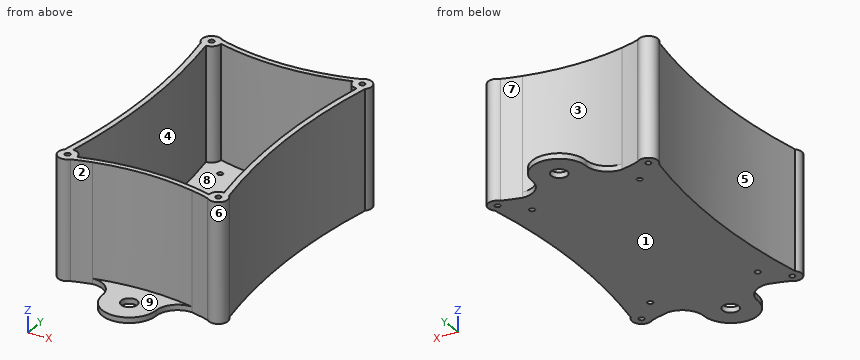
from build123d import *

# Parameters (mm, degrees)
F0_R     = 1
F1_DEPTH = 44
F0_R_2   = 3
F2_DEPTH = 2


with BuildPart() as f1:
    # F0 (on Top) → F1 (new body)
    with BuildSketch(Plane.XY):
        with BuildLine():
            ThreePointArc((-77.468398, 50.197146), (-73.493525, 8.17202), (-77.468398, -33.853106))
            ThreePointArc((-77.468398, -33.853106), (-77.468398, -38.802854), (-72.518651, -38.802854))
            ThreePointArc((-72.518651, -38.802854), (-68.996757, -37.763021), (-65.432755, -36.878214))
            ThreePointArc((-65.432755, -36.878214), (-46.993525, -34.82798), (-28.554295, -36.878214))
            ThreePointArc((-28.554295, -36.878214), (-24.990293, -37.763021), (-21.468398, -38.802854))
            ThreePointArc((-21.468398, -38.802854), (-16.518651, -38.802854), (-16.518651, -33.853106))
            ThreePointArc((-16.518651, -33.853106), (-20.493525, 8.17202), (-16.518651, 50.197146))
            ThreePointArc((-16.518651, 50.197146), (-16.518651, 55.146894), (-21.468398, 55.146894))
            ThreePointArc((-21.468398, 55.146894), (-24.990293, 54.10706), (-28.554295, 53.222254))
            ThreePointArc((-28.554295, 53.222254), (-46.993525, 51.17202), (-65.432755, 53.222254))
            ThreePointArc((-65.432755, 53.222254), (-68.996757, 54.10706), (-72.518651, 55.146894))
            ThreePointArc((-72.518651, 55.146894), (-77.468398, 55.146894), (-77.468398, 50.197146))
        make_face()
        with Locations((-74.993525, -36.32798)):
            Circle(F0_R, mode=Mode.SUBTRACT)
        with Locations((-18.993525, -36.32798)):
            Circle(F0_R, mode=Mode.SUBTRACT)
        with BuildLine():
            ThreePointArc((-74.993525, 49.17202), (-72.518651, 50.197146), (-71.493525, 52.67202))
            ThreePointArc((-71.493525, 52.67202), (-46.993525, 49.17202), (-22.493525, 52.67202))
            ThreePointArc((-22.493525, 52.67202), (-21.468398, 50.197146), (-18.993525, 49.17202))
            ThreePointArc((-18.993525, 49.17202), (-22.493525, 8.17202), (-18.993525, -32.82798))
            ThreePointArc((-18.993525, -32.82798), (-21.468398, -33.853106), (-22.493525, -36.32798))
            ThreePointArc((-22.493525, -36.32798), (-46.993525, -32.82798), (-71.493525, -36.32798))
            ThreePointArc((-71.493525, -36.32798), (-72.518651, -33.853106), (-74.993525, -32.82798))
            ThreePointArc((-74.993525, -32.82798), (-71.493525, 8.17202), (-74.993525, 49.17202))
        make_face(mode=Mode.SUBTRACT)
        with Locations((-74.993525, 52.67202)):
            Circle(F0_R, mode=Mode.SUBTRACT)
        with Locations((-18.993525, 52.67202)):
            Circle(F0_R, mode=Mode.SUBTRACT)
    extrude(amount=F1_DEPTH)

    # F0 (on Top) → F2 (join)
    with BuildSketch(Plane.XY):
        with BuildLine():
            ThreePointArc((-28.554295, -36.878214), (-46.993525, -34.82798), (-65.432755, -36.878214))
            ThreePointArc((-65.432755, -36.878214), (-59.507969, -39.04294), (-56.993525, -44.82798))
            ThreePointArc((-56.993525, -44.82798), (-46.993525, -54.82798), (-36.993525, -44.82798))
            ThreePointArc((-36.993525, -44.82798), (-34.47908, -39.04294), (-28.554295, -36.878214))
        make_face()
        with Locations((-46.993525, -44.82798)):
            Circle(F0_R_2, mode=Mode.SUBTRACT)
        with BuildLine():
            ThreePointArc((-56.993525, 61.17202), (-59.507969, 55.38698), (-65.432755, 53.222254))
            ThreePointArc((-65.432755, 53.222254), (-46.993525, 51.17202), (-28.554295, 53.222254))
            ThreePointArc((-28.554295, 53.222254), (-34.47908, 55.38698), (-36.993525, 61.17202))
            ThreePointArc((-36.993525, 61.17202), (-46.993525, 71.17202), (-56.993525, 61.17202))
        make_face()
        with Locations((-46.993525, 61.17202)):
            Circle(F0_R_2, mode=Mode.SUBTRACT)
        with BuildLine():
            ThreePointArc((-22.493525, 52.67202), (-46.993525, 49.17202), (-71.493525, 52.67202))
            ThreePointArc((-71.493525, 52.67202), (-72.518651, 50.197146), (-74.993525, 49.17202))
            ThreePointArc((-74.993525, 49.17202), (-71.493525, 8.17202), (-74.993525, -32.82798))
            ThreePointArc((-74.993525, -32.82798), (-72.518651, -33.853106), (-71.493525, -36.32798))
            ThreePointArc((-71.493525, -36.32798), (-46.993525, -32.82798), (-22.493525, -36.32798))
            ThreePointArc((-22.493525, -36.32798), (-21.468398, -33.853106), (-18.993525, -32.82798))
            ThreePointArc((-18.993525, -32.82798), (-22.493525, 8.17202), (-18.993525, 49.17202))
            ThreePointArc((-18.993525, 49.17202), (-21.468398, 50.197146), (-22.493525, 52.67202))
        make_face()
        with Locations((-66.993525, -28.32798)):
            Circle(F0_R, mode=Mode.SUBTRACT)
        with Locations((-26.993525, -28.32798)):
            Circle(F0_R, mode=Mode.SUBTRACT)
        with Locations((-66.993525, 44.67202)):
            Circle(F0_R, mode=Mode.SUBTRACT)
        with Locations((-26.993525, 44.67202)):
            Circle(F0_R, mode=Mode.SUBTRACT)
    extrude(amount=F2_DEPTH)


solid = f1.part
Source: CAD feature listing. Evaluate the final solid. Frame: model axes, mm. Face numbers are marked on the shaded views. A direction names the side the tool comes from. Round coordinates to 2 decimals unless told otherwise and drop trailing zeros. Loops run counter-clockwise (first coordinate to the right, second up) from the corner with the lowest first, then second, coordinate; pieces in that order, holes last. Notation, with made-up numbers: (65, 12) - (69, 12) arc R37 ccw to (69, 48) - close; hole circle Ø8 at (83.5, 35). An arc over 180 degrees is marked (long way). Write item = value, one per line. Start each with the question number.
Item 1: Section query C-C on y = 1.5. Output: boundary loops of the cut face in (x, z), plus the area to 3 significant figures.
Item 2: First-contact query: pin 1 Ø1 at (x, z) = (-34, 39) entering from -Y; pin 2 Ø10 at (x, z) = (-48.5, 32) entering from +Y; pin 3 Ø5 at (x, z) = (-25.5, 32) entering from -Y. Flat tips, straight axial feed; report the tip coordinate or a pass-through.
Item 3: Section query D-D on x = -39. Output: boundary loops of the cut face in (y, z), plus the area to 3 significant figures.
Item 4: Mould query, pull axis Y, two halves, no side actions, for the marked faces 1, 2, 3 and 4. Classes: released by +Y, released by -Y, zero draft, split by the parting line, or undercut.
Item 5: Reachability of the marked faces 5, 6, 7, 8 and 9 from +Z, -Z, +X, -X, +Y, -Y: full face, straight path, thin tool, end or side. Return the list, or none.
Item 6: Section query B-B on z = 16.5. Output: boundary loops of the cut face in (x, y), plus the area to 3 significant figures.
Item 7: Section query A-A on x = -47. Output: boundary loops of the cut face in (y, z), plus the area to 3 significant figures.
Item 8: Material intervals for line 1 (Y direction, x = -46.5, z = 21.5); line 2 (X direction, y = 9, z = 9.5); line 3 (Z direction, x = -52.5, y = 27.5), sorted ascending.
Results list:
q1.outline = (-73.59, 0) - (-20.39, 0) - (-20.39, 44) - (-22.4, 44) - (-22.4, 2) - (-71.59, 2) - (-71.59, 44) - (-73.59, 44) - close
q1.area = 275 mm²
q2.pin_1 = -35.92
q2.pin_2 = 51.42
q2.pin_3 = -38.33
q3.outline = (-50.84, 0) - (67.18, 0) - (67.18, 2) - (51.55, 2) - (51.55, 44) - (49.54, 44) - (49.54, 2) - (-33.19, 2) - (-33.19, 44) - (-35.21, 44) - (-35.21, 2) - (-50.84, 2) - close
q3.area = 405 mm²
q4.face_1 = zero draft
q4.face_2 = released by -Y
q4.face_3 = released by +Y
q4.face_4 = undercut
q5.face_5 = +Z, -Z, -X
q5.face_6 = +Z, -Z
q5.face_7 = +Z, -Z, +Y
q5.face_8 = +Z
q5.face_9 = +Z, -Y
q6.outline = (-77.47, -33.85) arc R3.5 ccw to (-72.52, -38.8) arc R83.94 cw to (-65.43, -36.88) arc R83.94 cw to (-28.55, -36.88) arc R83.94 cw to (-21.47, -38.8) arc R3.5 ccw to (-16.52, -33.85) arc R224.15 cw to (-16.52, 50.2) arc R3.5 ccw to (-21.47, 55.15) arc R83.94 cw to (-28.55, 53.22) arc R83.94 cw to (-65.43, 53.22) arc R83.94 cw to (-72.52, 55.15) arc R3.5 ccw to (-77.47, 50.2) arc R224.15 cw to start; hole circle Ø2 at (-74.99, -36.33); hole circle Ø2 at (-74.99, 52.67); hole (-74.99, -32.83) arc R3.5 cw to (-71.49, -36.33) arc R87.5 cw to (-22.49, -36.33) arc R3.5 cw to (-18.99, -32.83) arc R241.89 cw to (-18.99, 49.17) arc R3.5 cw to (-22.49, 52.67) arc R87.5 cw to (-71.49, 52.67) arc R3.5 cw to (-74.99, 49.17) arc R241.89 cw to start; hole circle Ø2 at (-18.99, -36.33); hole circle Ø2 at (-18.99, 52.67)
q6.area = 691 mm²
q7.outline = (-54.83, 0) - (-47.83, 0) - (-47.83, 2) - (-54.83, 2) - close; (-41.83, 0) - (58.17, 0) - (58.17, 2) - (51.17, 2) - (51.17, 44) - (49.17, 44) - (49.17, 2) - (-32.83, 2) - (-32.83, 44) - (-34.83, 44) - (-34.83, 2) - (-41.83, 2) - close; (64.17, 0) - (71.17, 0) - (71.17, 2) - (64.17, 2) - close
q7.area = 396 mm²
q8.line_1 = -34.83 to -32.83, 49.17 to 51.17
q8.line_2 = -73.5 to -71.49, -22.49 to -20.49
q8.line_3 = 0 to 2
